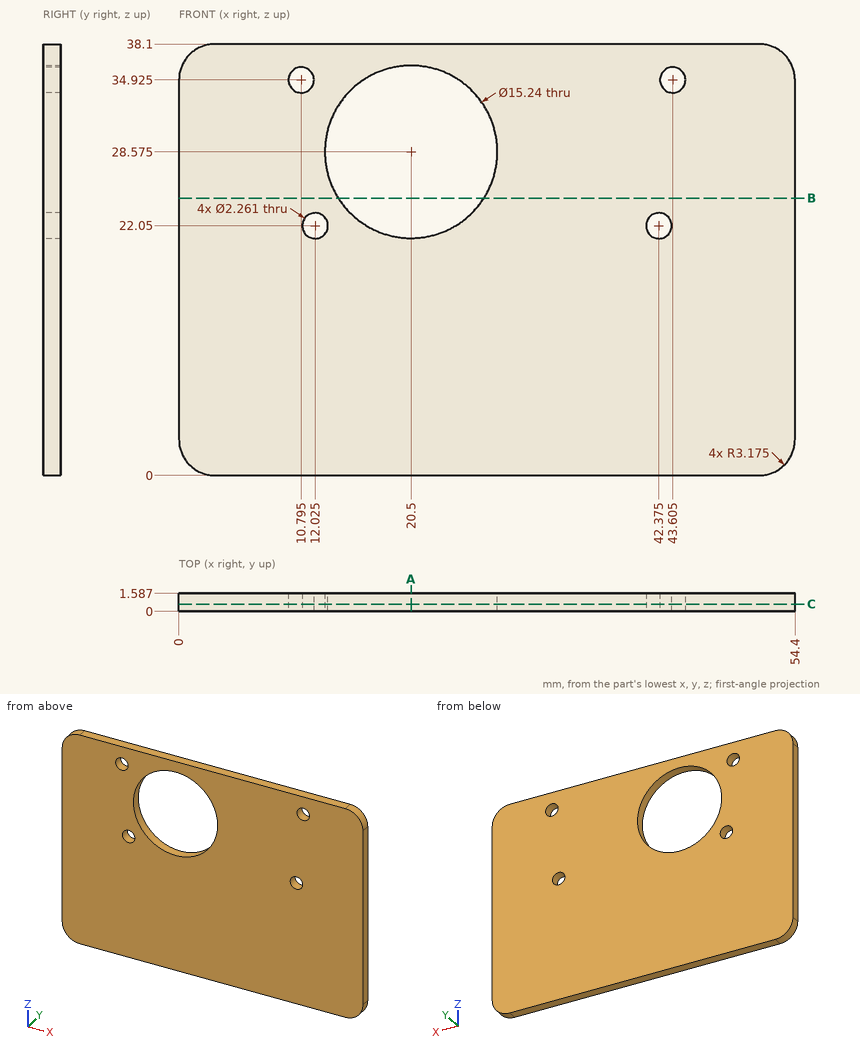
Geometry check sheet. Reference: drawing and pictorial views, mm from the part's lowest x, y, z. Coordinates: 2 decimals unless noted, no trailing zeros. Loops run counter-clockwise (first coordinate to the right, second up) from the corner with the lowest first, then second, coordinate; pieces in that order, holes last. Notation, with made-up numbers: (49, 79) -> (54, 79) arc R24 ccw to (54, 117) -> close; hole circle Ø3 at (31, 31). An arc over 180 degrees is marked (long way). Write item = value, one per line. Start each with the question number.
1. Section check B-B on z = 24.5. Record the cut outline in (x, y).
2. Section check A-A on x = 20.5. Record the cut outline in (y, z) (1 decimal).
3. Depth check by flat-ended pin: P1, Ø13.5, axis at x = 20.5, z = 28.575, coming from the +Y side. Enter the tip coordinate at first touch or a pass-through.
4. Section check C-C on y = 0.65. Give the number of separate pieces and of enclosed holes in the cut face, then the cut area to 3 significant figures.
5. Material ranges on line 1 (Z direction, x = 12, y = 0.9); line 2 (X direction, y = 0.65, z = 29); line 3 (X direction, y = 1, z = 35) (1 decimal), recorded low to high.
Responses:
q1.outline = (0, 0) -> (14.06, 0) -> (14.06, 1.59) -> (0, 1.59) -> close; (26.94, 0) -> (54.4, 0) -> (54.4, 1.59) -> (26.94, 1.59) -> close
q2.outline = (0, 0) -> (1.6, 0) -> (1.6, 21) -> (0, 21) -> close; (0, 36.2) -> (1.6, 36.2) -> (1.6, 38.1) -> (0, 38.1) -> close
q3.P1 = through
q4.separate_pieces = 1
q4.enclosed_holes = 5
q4.area = 1,870 mm2
q5.line_1 = 0 to 20.92, 23.18 to 38.1
q5.line_2 = 0 to 12.89, 28.11 to 54.4
q5.line_3 = 0 to 9.7, 11.9 to 16.4, 24.6 to 42.5, 44.7 to 54.4
